from build123d import *

# Parameters (mm, degrees)
SKETCH_1_R          = 7.9
EXTRUDE_1_DEPTH     = 20
SKETCH_3_R          = 10
EXTRUDE_2_DEPTH     = 2
EXTRUDE_3_DEPTH     = 15
SKETCH_5_R          = 3.1
CUT_EXTRUDE_1_DEPTH = 10
CHAMFER_1_SIZE      = 0.5
SKETCH_6_R          = 2.6
CUT_EXTRUDE_2_DEPTH = 15
CHAMFER_2_SIZE      = 1


with BuildPart() as part:
    # 草图1 → 凸台-拉伸1 (new body)
    with BuildSketch(Plane(origin=(0, 0, 0), x_dir=(0, 0, -1), z_dir=(1, 0, 0))):
        Circle(SKETCH_1_R)
    extrude(amount=EXTRUDE_1_DEPTH)

    # 草图3 → 凸台-拉伸2 (add)
    with BuildSketch(Plane.ZY):
        Circle(SKETCH_3_R)
    extrude(amount=EXTRUDE_2_DEPTH)

    # 草图4 → 凸台-拉伸3 (add)
    with BuildSketch(Plane.ZY.offset(2)):
        Polygon((6.35, 3.666174209), (0, 7.332348419), (-6.35, 3.666174209), (-6.35, -3.666174209), (0, -7.332348419), (6.35, -3.666174209), align=None)
    extrude(amount=EXTRUDE_3_DEPTH)

    # 草图5 → 切除-拉伸1 (cut, symmetric)
    with BuildSketch(Plane(origin=(0, 0, 0), x_dir=(1, 0, 0), z_dir=(0, 1, 0))):
        with Locations((10, 0)):
            Circle(SKETCH_5_R)
    extrude(amount=CUT_EXTRUDE_1_DEPTH, both=True, mode=Mode.SUBTRACT)

    # 倒角1
    chamfer_1_edges = [part.edges().sort_by_distance(p)[0] for p in [
        (-2, 0, -10),
    ]]
    chamfer(chamfer_1_edges, length=CHAMFER_1_SIZE)

    # 草图6 → 切除-拉伸2 (cut)
    with BuildSketch(Plane.ZY.offset(17)):
        Circle(SKETCH_6_R)
    extrude(amount=-CUT_EXTRUDE_2_DEPTH, mode=Mode.SUBTRACT)

    # 倒角2
    chamfer_2_edges = [part.edges().sort_by_distance(p)[0] for p in [
        (20, 0, 7.9),
    ]]
    chamfer(chamfer_2_edges, length=CHAMFER_2_SIZE)


solid = part.part
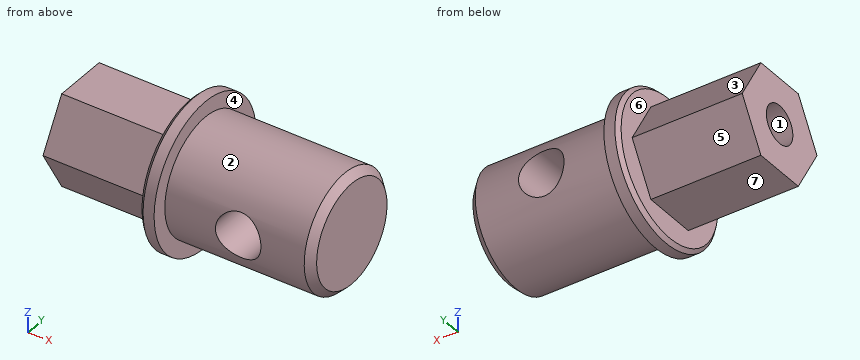
Here's how the part is built. I have some questions about the finished solid (model axes, mm). Face numbers are marked on the shaded views. A direction names the side the tool comes from. Coordinates: 2 decimals unless noted, no trailing zeros. Write each loop counter-clockwise with the first axis right and the second up, starting at its lowest first coordinate (ties: lowest second). Pieces come first, ordered by that corner, then holes.
1) If I drill on line 1 (Y direction, x = -6.75, z = 0); line 2 (X direction, y = -6, z = -5.25); line 3 (Z direction, x = -10.5, y = -0.25), over which ranges is the centre line in solid material (lowest first)?
Filled in:
line 1: y = -7.33 to -2.6, 2.6 to 7.33
line 2: x = -2 to 0
line 3: z = -6.35 to -2.59, 2.59 to 6.35
2) Thinking about a two-plate mould opening in Y: for the marked faces 1, 2, 3 and 4, which applies, +Y half, -Y half, draft (parallel to the pull), parting line (faces both ways), or undercut?
Filled in:
face 1: undercut
face 2: parting line
face 3: +Y half
face 4: draft
3) Which directions (+Z, -Z, +X, -X, +Y, -Y) give clear straight access to the entire face, cutting with the end or side of a thin tool? Please do the marked faces 5, 6 and 7.
Filled in:
face 5: -Z, -X, +Y
face 6: -X
face 7: -Z, -X, +Y, -Y
4) If we section it at B-B (x = 10): List the corners of the cut face in (y, z) for me.
Filled in:
outline: (-7.27, -3.1) arc R7.9 ccw to (7.27, -3.1) - close; (-7.27, 3.1) - (7.27, 3.1) arc R7.9 ccw to start
5) I'm going to push flat-ended pins straight in: pin 1 (4 mm diameter, centred on x = -3.5, z = -2.5, fed in from +Y); pin 2 (4 mm diameter, centred on y = -7.5, z = 3, fed in from +X); pin 3 (6 mm diameter, centred on x = 0, y = -4, fed in from +Z); pin 4 (8 mm diameter, centred on x = -8.5, y = 4, fed in from -Z). Where does each tip first touch, or does it pass through?
Filled in:
pin 1: stops at y = 9.74
pin 2: stops at x = 20
pin 3: stops at z = 9.95
pin 4: stops at z = -6.35
6) If we section it at C-C (x = 4.5): List the corners of the cut face in (y, z) for me.
Filled in:
outline: circle Ø15.8 at (0, 0)
7) If we section it at A-A (y = 0): List the corners of the cut face in (x, z) for me, plus the area to 3 significant figures.
Filled in:
outline: (-17, -6.35) - (-2, -6.35) - (-2, -9.5) - (-1.5, -10) - (0, -10) - (0, -7.9) - (19, -7.9) - (20, -6.9) - (20, 6.9) - (19, 7.9) - (0, 7.9) - (0, 10) - (-1.5, 10) - (-2, 9.5) - (-2, 6.35) - (-17, 6.35) - (-17, 2.6) - (-2, 2.6) - (-2, -2.6) - (-17, -2.6) - close; hole circle Ø6.2 at (10, 0)
area: 437 mm2
